Can you work these out from the model? Positions are in its coordinate system, mm. Face numbers are marked on the shaded views. A direction names the side the tool comes from. Give positions to 0.01 mm unless a question says otherwise; leave off trailing zeros. Order: outer loops, then holes, each group sorted by start corner. A loop starts at its lowest first (then second) coordinate and runs counter-clockwise, first axis right, second up. Notation, with made-up numbers: (-19.75, 83) - (27.25, 83) arc R29 ccw to (27.25, 107) - close; hole circle Ø1 at (84, 77.25). An arc over 180 degrees is marked (long way). Answer as a JSON object with one key per item and string values.
```python
from build123d import *

# Parameters (mm, degrees)
SKETCH_1_W               = 65
SKETCH_1_H               = 15
EXTRUDE_1_DEPTH          = 2
SKETCH_2_R               = 1.25
SKETCH_2_R_2             = 3.45
SKETCH_2_R_3             = 1.5
SKETCH_2_R_4             = 1
CUT_EXTRUDE_1_DEPTH      = 2
SKETCH_4_R               = 1.5
EXTRUDE_2_DEPTH          = 2
SKETCH_5_R               = 7.5
SKETCH_5_R_2             = 7.2
EXTRUDE_3_DEPTH          = 6
SKETCH_5_8_R             = 1.25
SKETCH_5_8_R_2           = 7.2
EXTRUDE_4_DEPTH          = 6
CUT_EXTRUDE_2_DEPTH      = 3.5
CUT_EXTRUDE_2_DEPTH_BACK = 42.548164821
SKETCH_5_11_R            = 1.25
SKETCH_5_11_R_2          = 7.2
SKETCH_2_3_R             = 1.5
SKETCH_2_3_R_2           = 1
CUT_EXTRUDE_3_DEPTH      = 8


with BuildPart() as part:
    # 草图1 → 凸台-拉伸1 (new body)
    with BuildSketch(Plane(origin=(0, 0, 0), x_dir=(1, 0, 0), z_dir=(0, 1, 0))):
        with Locations((-7.5, 0)):
            Rectangle(SKETCH_1_W, SKETCH_1_H)
    extrude(amount=EXTRUDE_1_DEPTH)

    # 草图2 → 切除-拉伸1 (cut)
    with BuildSketch(Plane(origin=(0, 0, 0), x_dir=(1, 0, 0), z_dir=(0, 1, 0))):
        with Locations(Location((0, 0, 0), (0, 0, 270))):
            Circle(SKETCH_2_R)
        with Locations(Location((-16, 0, 0), (0, 0, 90))):
            Circle(SKETCH_2_R_2)
        with Locations(Location((-32, 0, 0), (0, 0, 270))):
            Circle(SKETCH_2_R_3)
        with Locations(Location((-26.5, 0, 0), (0, 0, 270))):
            Circle(SKETCH_2_R_4)
        with Locations(Location((-32, -5.5, 0), (0, 0, 270))):
            Circle(SKETCH_2_R_4)
        with Locations(Location((-37.5, 0, 0), (0, 0, 270))):
            Circle(SKETCH_2_R_4)
        with Locations(Location((-32, 5.5, 0), (0, 0, 270))):
            Circle(SKETCH_2_R_4)
    extrude(amount=CUT_EXTRUDE_1_DEPTH, mode=Mode.SUBTRACT)

    # 草图4 → 凸台-拉伸2 (add)
    with BuildSketch(Plane.XY.offset(7.5)):
        with Locations(Location((20, 1, 0), (0, 0, 221.810314896))):
            Circle(SKETCH_4_R)
        with Locations(Location((-20, 1, 0), (0, 0, 221.810314896))):
            Circle(SKETCH_4_R)
    extrude(amount=EXTRUDE_2_DEPTH)

    # 草图5 → 凸台-拉伸3 (add)
    # profile 1 of 2: a face of its own
    with BuildSketch(Plane(origin=(0, 2, 0), x_dir=(1, 0, 0), z_dir=(0, 1, 0))):
        with Locations(Location((-32, 0, 0), (0, 0, 270))):
            Circle(SKETCH_5_R)
        with Locations(Location((-32, 0, 0), (0, 0, 270))):
            Circle(SKETCH_5_R_2, mode=Mode.SUBTRACT)
    # profile 2 of 2: a face of its own
    with BuildSketch(Plane(origin=(0, 2, 0), x_dir=(1, 0, 0), z_dir=(0, 1, 0))):
        with BuildLine():
            Line((5.149029035, -6.7), (-5.149029035, -6.7))
            ThreePointArc((-5.149029035, -6.7), (-8.45, 0), (-5.149029035, 6.7))
            Line((-5.149029035, 6.7), (5.149029035, 6.7))
            ThreePointArc((5.149029035, 6.7), (8.45, 0), (5.149029035, -6.7))
        make_face()
        with BuildLine():
            Line((4.905354218, -6), (-4.905354218, -6))
            ThreePointArc((-4.905354218, -6), (-7.75, 0), (-4.905354218, 6))
            Line((-4.905354218, 6), (4.905354218, 6))
            ThreePointArc((4.905354218, 6), (7.75, 0), (4.905354218, -6))
        make_face(mode=Mode.SUBTRACT)
    extrude(amount=EXTRUDE_3_DEPTH)

    # 草图5<8> → 凸台-拉伸4 (add)
    # profile 1 of 2: a face of its own
    with BuildSketch(Plane(origin=(0, 2, 0), x_dir=(1, 0, 0), z_dir=(0, 1, 0))):
        with BuildLine():
            Line((4.905354218, -6), (-4.905354218, -6))
            ThreePointArc((-4.905354218, -6), (-7.75, 0), (-4.905354218, 6))
            Line((-4.905354218, 6), (4.905354218, 6))
            ThreePointArc((4.905354218, 6), (7.75, 0), (4.905354218, -6))
        make_face()
        with Locations(Location((0, 0, 0), (0, 0, 270))):
            Circle(SKETCH_5_8_R, mode=Mode.SUBTRACT)
    # profile 2 of 2: a face of its own
    with BuildSketch(Plane(origin=(0, 2, 0), x_dir=(1, 0, 0), z_dir=(0, 1, 0))):
        with Locations((-32, 0)):
            Circle(SKETCH_5_8_R_2)
    extrude(amount=EXTRUDE_4_DEPTH)

    # 草图5<11> → 切除-拉伸2 (cut, two sides: drawn at the far end of the back side and taken through both)
    # profile 1 of 2: a face of its own
    with BuildSketch(Plane(origin=(0, 2, 0), x_dir=(1, 0, 0), z_dir=(0, 1, 0)).offset(-CUT_EXTRUDE_2_DEPTH_BACK)):
        with BuildLine():
            Line((4.905354218, -6), (-4.905354218, -6))
            ThreePointArc((-4.905354218, -6), (-7.75, 0), (-4.905354218, 6))
            Line((-4.905354218, 6), (4.905354218, 6))
            ThreePointArc((4.905354218, 6), (7.75, 0), (4.905354218, -6))
        make_face()
        with Locations(Location((0, 0, 0), (0, 0, 270))):
            Circle(SKETCH_5_11_R, mode=Mode.SUBTRACT)
    # profile 2 of 2: a face of its own
    with BuildSketch(Plane(origin=(0, 2, 0), x_dir=(1, 0, 0), z_dir=(0, 1, 0)).offset(-CUT_EXTRUDE_2_DEPTH_BACK)):
        with Locations(Location((-32, 0, 0), (0, 0, 270))):
            Circle(SKETCH_5_11_R_2)
    extrude(amount=CUT_EXTRUDE_2_DEPTH + CUT_EXTRUDE_2_DEPTH_BACK, mode=Mode.SUBTRACT)

    # 草图2<3> → 切除-拉伸3 (cut)
    with BuildSketch(Plane(origin=(0, 0, 0), x_dir=(1, 0, 0), z_dir=(0, 1, 0))):
        with Locations(Location((-32, 0, 0), (0, 0, 270))):
            Circle(SKETCH_2_3_R)
        with Locations(Location((-32, 5.5, 0), (0, 0, 270))):
            Circle(SKETCH_2_3_R_2)
        with Locations(Location((-37.5, 0, 0), (0, 0, 270))):
            Circle(SKETCH_2_3_R_2)
        with Locations(Location((-32, -5.5, 0), (0, 0, 270))):
            Circle(SKETCH_2_3_R_2)
        with Locations(Location((-26.5, 0, 0), (0, 0, 270))):
            Circle(SKETCH_2_3_R_2)
    extrude(amount=CUT_EXTRUDE_3_DEPTH, mode=Mode.SUBTRACT)


solid = part.part
```
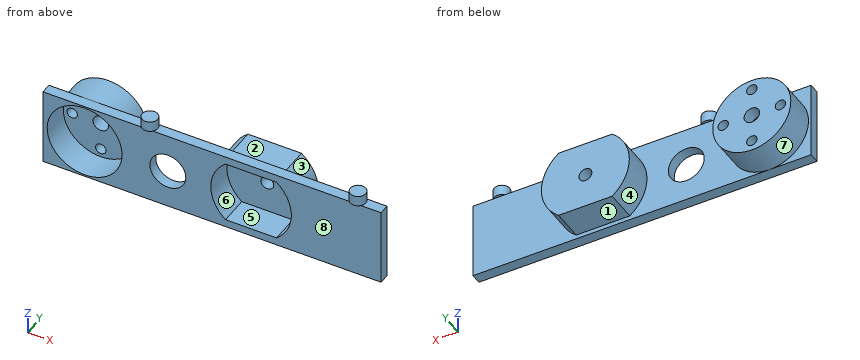
Q1. If we section it at D-D, the plane z = 0: Count the separate pieces of the cut face and the enclosed holes in it, then the cut area to 3 significant figures.
Recorded:
{"separate pieces": "6", "enclosed holes": "0", "area": "119 mm^2"}
Q2. If we section it at A-A, the plane y = 6.5: Please give me the cut outline in (x, z).
Recorded:
{"outline": "circle Ø15 at (-32, 0); (-5.15, -6.7) - (5.15, -6.7) arc R8.45 ccw to (5.15, 6.7) - (-5.15, 6.7) arc R8.45 ccw to start; hole circle Ø2 at (-37.5, 0); hole circle Ø3 at (-32, 0); hole circle Ø2 at (-32, -5.5); hole circle Ø2 at (-32, 5.5); hole circle Ø2 at (-26.5, 0); hole circle Ø2.5 at (0, 0)"}
Q3. We'd pull the mould along Z, two halves only. Please class the marked faces 6, 7 and 8: released by +Z, released by -Z, zero draft, split by the parting line, or undercut.
Recorded:
{"face 6": "undercut", "face 7": "split by the parting line", "face 8": "zero draft"}
Q4. If we section it at B-B, the plane y = 1: Please give me the cut outline in (x, z), then the cut area to 3 significant figures.
Recorded:
{"outline": "(-40, -7.5) - (25, -7.5) - (25, 7.5) - (21.5, 7.5) - (21.5, 9.5) - (18.5, 9.5) - (18.5, 7.5) - (-18.5, 7.5) - (-18.5, 9.5) - (-21.5, 9.5) - (-21.5, 7.5) - (-40, 7.5) - close; hole circle Ø14.4 at (-32, 0); hole circle Ø6.9 at (-16, 0); hole (-4.91, -6) - (4.91, -6) arc R7.75 ccw to (4.91, 6) - (-4.91, 6) arc R7.75 ccw to start", "area": "622 mm^2"}
Q5. I need wall thicknesses on L1, parallel to Z at x = -0.5, y = 4.5; L2, parallel to X at y = 5, z = -0.75; L3, parallel to Z at x = -32, y = 1.6. Which ranges of each line are inside material? Lowest first, please.
Recorded:
{"L1": "z = -6.7 to -6, 6 to 6.7", "L2": "x = -39.46 to -39.16, -24.84 to -24.54, -8.42 to -7.71, 7.71 to 8.42", "L3": "z = -7.5 to -7.2, 7.2 to 7.5"}
Q6. Which directions (+Z, -Z, +X, -X, +Y, -Y) give clear straight access to the entire face, cutting with the end or side of a thin tool? Please do the marked faces 1, 2, 3, 4 and 5.
Recorded:
{"face 1": "-Z, +X, +Y", "face 2": "+Z, +X, +Y", "face 3": "+X, +Y", "face 4": "+Y", "face 5": "-Y"}
Q7. I'm going to push flat-ended pins straight in: pin 1 Ø3 at (x, z) = (0, 0) entering from -Y; pin 2 Ø4 at (x, z) = (15, 3) entering from +Y; pin 3 Ø5.5 at (x, z) = (-16, 0) entering from -Y; pin 4 Ø3 at (x, y) = (2, 4) entering from +Z. Where does each tip first touch, or does it pass through?
Recorded:
{"pin 1": "stops at y = 5.5", "pin 2": "stops at y = 2", "pin 3": "passes through", "pin 4": "stops at z = 6.7"}
Q8. If we section it at C-C, the plane x = -20: Please give me the cut outline in (y, z).
Recorded:
{"outline": "(-0.5, 7.5) - (0, 7.5) - (0, -7.5) - (2, -7.5) - (2, 7.5) - (2.5, 7.5) - (2.5, 9.5) - (-0.5, 9.5) - close"}
